The listing builds one solid part. Answer for the finished solid, in the listing's coordinates (mm). A direction names the side the tool comes from. Give positions to 0.01 mm unless a question says otherwise; leave off trailing zeros. Write each loop counter-clockwise with the first axis right and the second up, starting at its lowest first coordinate (ties: lowest second). Pieces come first, ordered by that corner, then holes. Notation, with made-up numbers: (-7, -29) -> (38, -29) arc R22 ccw to (38, -16) -> close; hole circle Ø9 at (28.5, 11). An arc over 180 degrees is marked (long way). Put each result on its own line as item: value. Start each with the question number.
1) A cutting plane is placed at A-A (x = 5). Write down the section's boundary in (y, z), then the cut area to 3 significant figures.
2) For a pull along Z with two mould halves and no side action, classify faces 6 (the flat face through (3, 1, -5)), 7 (the flat face through (3, 1, -25)), 8 (the flat face through (19.5, 1, -20)) as released by +Z, released by -Z, zero draft, split by the parting line, or undercut.
3) A cutting plane is placed at B-B (y = 0.7). Give the number of separate pieces and of enclosed holes in the cut face, then the cut area to 3 significant figures.
4) For faces 1 (the flat face through (5.5, 1, -2)), 2 (the flat face through (0, 1, -10)), 3 (the flat face through (12, 1, 0)), 4 (the flat face through (5.5, 1, -37)), 5 (the flat face through (5.5, 1, -20)), determine the directions among +Z, -Z, +X, -X, +Y, -Y from which every point of the face is accessible in a straight line to the end or side of a thin tool.
5) A cutting plane is placed at C-C (z = -16.5). Write down the section's boundary in (x, y), then the cut area to 3 significant figures.
6) Flat-ended cylindrical pins translate along their axes: pin 1 Ø0.8 at (y, z) = (1, -2) entering from -X; pin 2 Ø0.5 at (x, y) = (3, 0.5) entering from -Z. Find the tip coordinate at first contact, or state that the pin passes through.
7) Find the intervals of material crossed by line 1 along Z through (x, y) = (13.5, 0.95); line 2 along X through (y, z) = (0.4, -25.4); line 3 along X through (y, z) = (0.85, -20), in increasing order. Write a range as from..to.
from build123d import *

# Parameters (mm, degrees)
SKETCH_1_W                  = 19.5
SKETCH_1_H                  = 40
EXTRUDE_1_DEPTH             = 1.6
SKETCH_2_W                  = 5.5
SKETCH_2_H                  = 5
SKETCH_2_H_2                = 10
CUT_EXTRUDE_1_DEPTH         = 45.528754755
HOLE_WIZARD_0_5_0_5_1_D     = 0.5
PATTERN_LINEAR_1_COUNT      = 4
PATTERN_LINEAR_1_PITCH      = 2.5
HOLE_WIZARD_0_5_0_5_2_D     = 0.5
PATTERN_LINEAR_2_COUNT      = 3
PATTERN_LINEAR_2_PITCH      = 2.54
PATTERN_LINEAR_2_COUNT_DIR2 = 9
PATTERN_LINEAR_2_PITCH_DIR2 = 2.7
HOLE_WIZARD_0_5_0_5_3_D     = 0.5
PATTERN_LINEAR_3_COUNT      = 2
PATTERN_LINEAR_3_PITCH      = 2.54
HOLE_WIZARD_0_5_0_5_4_D     = 0.5
PATTERN_LINEAR_4_COUNT      = 4
PATTERN_LINEAR_4_PITCH      = 2.5


with BuildPart() as part:
    # 스케치1 → 보스-돌출1 (new body)
    with BuildSketch(Plane(origin=(0, 0, 0), x_dir=(1, 0, 0), z_dir=(0, 1, 0))):
        with Locations((9.75, 20)):
            Rectangle(SKETCH_1_W, SKETCH_1_H)
    extrude(amount=EXTRUDE_1_DEPTH)

    # 스케치2 → 컷-돌출1 (cut, through all)
    with BuildSketch(Plane(origin=(0, 1.6, 0), x_dir=(1, 0, 0), z_dir=(0, 1, 0))):
        with Locations((2.75, 2.5)):
            Rectangle(SKETCH_2_W, SKETCH_2_H)
        with Locations((2.75, 37.5)):
            Rectangle(SKETCH_2_W, SKETCH_2_H)
        with Locations((2.75, 20)):
            Rectangle(SKETCH_2_W, SKETCH_2_H_2)
    extrude(amount=-CUT_EXTRUDE_1_DEPTH, mode=Mode.SUBTRACT)

    # Ø0.5 (0.5) 지름 구멍1 (through all)
    with Locations(Plane(origin=(0, 1.6, 0), x_dir=(1, 0, 0), z_dir=(0, 1, 0))):
        with Locations((8.5, 35.4)):
            hole_wizard_0_5_0_5_1 = Hole(HOLE_WIZARD_0_5_0_5_1_D / 2)

    # 선형 패턴1: Ø0.5 (0.5) 지름 구멍1 ×4
    with Locations(*[(i * PATTERN_LINEAR_1_PITCH, 0, 0) for i in range(1, PATTERN_LINEAR_1_COUNT)]):
        add(hole_wizard_0_5_0_5_1, mode=Mode.SUBTRACT)

    # Ø0.5 (0.5) 지름 구멍2 (through all)
    with Locations(Plane(origin=(0, 1.6, 0), x_dir=(1, 0, 0), z_dir=(0, 1, 0))):
        with Locations((7.27, 30.8)):
            hole_wizard_0_5_0_5_2 = Hole(HOLE_WIZARD_0_5_0_5_2_D / 2)

    # 선형 패턴2: Hole Wizard 0.5 _0.5_ _ _2 3 × 9
    with Locations(*[(i * PATTERN_LINEAR_2_PITCH, 0, j * PATTERN_LINEAR_2_PITCH_DIR2) for i in range(PATTERN_LINEAR_2_COUNT) for j in range(PATTERN_LINEAR_2_COUNT_DIR2) if (i, j) != (0, 0)]):
        add(hole_wizard_0_5_0_5_2, mode=Mode.SUBTRACT)

    # Ø0.5 (0.5) 지름 구멍3 (through all)
    with Locations(Plane(origin=(0, 1.6, 0), x_dir=(1, 0, 0), z_dir=(0, 1, 0))):
        with Locations((15.941577117, 10.725654996)):
            hole_wizard_0_5_0_5_3 = Hole(HOLE_WIZARD_0_5_0_5_3_D / 2)

    # 선형 패턴3: Ø0.5 (0.5) 지름 구멍3 ×2
    with Locations(*[(0, 0, -i * PATTERN_LINEAR_3_PITCH) for i in range(1, PATTERN_LINEAR_3_COUNT)]):
        add(hole_wizard_0_5_0_5_3, mode=Mode.SUBTRACT)

    # Ø0.5 (0.5) 지름 구멍4 (through all)
    with Locations(Plane(origin=(0, 1.6, 0), x_dir=(1, 0, 0), z_dir=(0, 1, 0))):
        with Locations((8.5, 3.4)):
            hole_wizard_0_5_0_5_4 = Hole(HOLE_WIZARD_0_5_0_5_4_D / 2)

    # 선형 패턴4: Ø0.5 (0.5) 지름 구멍4 ×4
    with Locations(*[(i * PATTERN_LINEAR_4_PITCH, 0, 0) for i in range(1, PATTERN_LINEAR_4_COUNT)]):
        add(hole_wizard_0_5_0_5_4, mode=Mode.SUBTRACT)


solid = part.part
Reply:
1. outline: (0, -35) -> (1.6, -35) -> (1.6, -25) -> (0, -25) -> close; (0, -15) -> (1.6, -15) -> (1.6, -5) -> (0, -5) -> close
1. area: 32.0 mm2
2. face 6: released by +Z
2. face 7: undercut
2. face 8: zero draft
3. separate pieces: 1
3. enclosed holes: 37
3. area: 663 mm2
4. face 1: +Z, -X, +Y, -Y
4. face 2: +Z, -Z, -X, +Y, -Y
4. face 3: +Z, +X, -X, +Y, -Y
4. face 4: -Z, -X, +Y, -Y
4. face 5: -X, +Y, -Y
5. outline: (5.5, 0) -> (19.5, 0) -> (19.5, 1.6) -> (5.5, 1.6) -> close
5. area: 22.4 mm2
6. pin 1: stops at x = 5.5
6. pin 2: stops at z = -35
7. line 1: z = -40..-35.65, -35.15..-3.65, -3.15..0
7. line 2: x = 0..7.02, 7.52..9.56, 10.06..12.1, 12.6..19.5
7. line 3: x = 5.5..7.02, 7.52..9.56, 10.06..12.1, 12.6..19.5
